from build123d import *

# Parameters (mm, degrees)
BLANKSKE_W               = 40
BLANKSKE_H               = 8.5
BLANK_DEPTH              = 10
TOOTHCUTSIM_DEPTH        = 43.09809972
TEETHCUTS_COUNT          = 14
TEETHCUTS_PITCH          = 3.14159265
BOSS_EXTRUDE1_DEPTH      = 10
SKETCH2_W                = 3
SKETCH2_H                = 3
BOSS_EXTRUDE2_DEPTH      = 60
CUT_EXTRUDE2_DEPTH       = 73.801098893
MOVE_FACE2_BY            = 5
FILLET2_R                = 8
SKETCH3_R                = 1.675
CUT_EXTRUDE1_DEPTH       = 69.738635424
SKETCH6_W                = 14.81
SKETCH6_H                = 5
BOSS_EXTRUDE3_DEPTH      = 2.5
SKETCH7_W                = 2.5
SKETCH7_H                = 5
BOSS_EXTRUDE4_DEPTH      = 5
M2_START                 = -34.81
M2_CLEARANCE_SLOT1_DEPTH = 2.5
BOSS_EXTRUDE5_DEPTH      = 5
FILLET3_R                = 5
FILLET4_R                = 1
FILLET5_R                = 0.25


with BuildPart() as part:
    # BlankSke → Blank (new body)
    with BuildSketch(Plane.XY):
        with Locations((20, 4.25)):
            Rectangle(BLANKSKE_W, BLANKSKE_H)
    extrude(amount=-BLANK_DEPTH)

    # TooCutSkeSim → ToothCutSim (cut, through all)
    with BuildSketch(Plane.XY):
        Polygon((0.44443537, 6.25), (-0.44443537, 6.25), (-1.272613241, 8.5254), (1.272613241, 8.5254), align=None)
    toothcutsim = extrude(amount=-TOOTHCUTSIM_DEPTH, mode=Mode.SUBTRACT)

    # TeethCuts: ToothCutSim ×14
    with Locations(*[(i * TEETHCUTS_PITCH, 0, 0) for i in range(1, TEETHCUTS_COUNT)]):
        add(toothcutsim, mode=Mode.SUBTRACT)

    # Sketch1 → Boss-Extrude1 (add)
    with BuildSketch(Plane.XY):
        Polygon((-20, 0), (-20, -40), (-10, -40), (-10, 0), (0, 0), (0, 6.25), (-20, 6.25), align=None)
    extrude(amount=-BOSS_EXTRUDE1_DEPTH)

    # Sketch2 → Boss-Extrude2 (add)
    with BuildSketch(Plane(origin=(40, 0, 0), x_dir=(0, 0, -1), z_dir=(1, 0, 0))):
        with Locations((-1.5, 3)):
            Rectangle(SKETCH2_W, SKETCH2_H)
    extrude(amount=-BOSS_EXTRUDE2_DEPTH)

    # Sketch5 → Cut-Extrude2 (cut, through all)
    with BuildSketch(Plane(origin=(40, 0, 0), x_dir=(0, 0, -1), z_dir=(1, 0, 0))):
        with BuildLine():
            Line((10, 2), (10, 4))
            Line((10, 4), (8, 4))
            ThreePointArc((8, 4), (7, 3), (8, 2))
            Line((8, 2), (10, 2))
        make_face()
    extrude(amount=-CUT_EXTRUDE2_DEPTH, mode=Mode.SUBTRACT)

    # Move Face2: a face moved inward by 5.0
    extrude(part.faces().sort_by_distance((-10, -20, -5))[0], amount=MOVE_FACE2_BY, dir=(-1, 0, 0), mode=Mode.SUBTRACT)

    # Fillet2
    fillet2_edges = [part.edges().sort_by_distance(p)[0] for p in [
        (-15, 0, -5),
    ]]
    fillet(fillet2_edges, radius=FILLET2_R)

    # Sketch3 → Cut-Extrude1 (cut, through all)
    with BuildSketch(Plane.ZY.offset(15)):
        with Locations((-5, -35)):
            Circle(SKETCH3_R)
    extrude(amount=CUT_EXTRUDE1_DEPTH, mode=Mode.SUBTRACT)

    # Sketch6 → Boss-Extrude3 (add)
    with BuildSketch(Plane(origin=(0, 0, -10), x_dir=(-1, 0, 0), z_dir=(0, 0, -1))):
        with Locations((27.405, -15.8)):
            Rectangle(SKETCH6_W, SKETCH6_H)
        Polygon((20, -40), (15, -40), (15, -46.25), (34.81, -46.25), (34.81, -41.25), (20, -41.25), align=None)
    extrude(amount=-BOSS_EXTRUDE3_DEPTH)

    # Sketch7 → Boss-Extrude4 (add)
    with BuildSketch(Plane.XY.offset(-7.5)):
        with Locations((-33.56, -15.8)):
            Rectangle(SKETCH7_W, SKETCH7_H)
        with Locations((-33.56, -43.75)):
            Rectangle(SKETCH7_W, SKETCH7_H)
    extrude(amount=BOSS_EXTRUDE4_DEPTH)

    # M2 Clearance Slot1: read off the stored shape, not the designer's step
    # M2 Clearance Slot1 outline → M2 Clearance Slot1 (cut)
    with BuildSketch(Plane.YZ.offset(M2_START)):
        with BuildLine():
            ThreePointArc((-44.25, -3.8), (-45.45, -5), (-44.25, -6.2))
            Line((-44.25, -6.2), (-43.25, -6.2))
            ThreePointArc((-43.25, -6.2), (-42.05, -5), (-43.25, -3.8))
            Line((-43.25, -3.8), (-44.25, -3.8))
        make_face()
        with BuildLine():
            ThreePointArc((-16.3, -3.8), (-17.5, -5), (-16.3, -6.2))
            Line((-16.3, -6.2), (-15.3, -6.2))
            ThreePointArc((-15.3, -6.2), (-14.1, -5), (-15.3, -3.8))
            Line((-15.3, -3.8), (-16.3, -3.8))
        make_face()
    extrude(amount=M2_CLEARANCE_SLOT1_DEPTH, mode=Mode.SUBTRACT)

    # M2 Clearance Slot1 2: loft between two sections, ruled curve by curve
    m2_clearance_slot1_2_from = [
        Edge.make_three_point_arc((-34.785, -43.25, -3.8), (-34.785, -42.401471863, -4.151471863), (-34.785, -42.05, -5)),
        Edge.make_three_point_arc((-34.785, -42.05, -5), (-34.785, -42.401471863, -5.848528137), (-34.785, -43.25, -6.2)),
        Edge.make_three_point_arc((-34.785, -44.25, -6.2), (-34.785, -45.098528137, -5.848528137), (-34.785, -45.45, -5)),
        Edge.make_three_point_arc((-34.785, -45.45, -5), (-34.785, -45.098528137, -4.151471863), (-34.785, -44.25, -3.8)),
        Edge.make_line((-34.785, -43.25, -6.2), (-34.785, -44.25, -6.2)),
        Edge.make_line((-34.785, -43.25, -3.8), (-34.785, -44.25, -3.8)),
    ]
    m2_clearance_slot1_2_to = [
        Edge.make_three_point_arc((-34.81, -43.25, -3.775), (-34.81, -42.383794193, -4.133794193), (-34.81, -42.025, -5)),
        Edge.make_three_point_arc((-34.81, -42.025, -5), (-34.81, -42.383794193, -5.866205807), (-34.81, -43.25, -6.225)),
        Edge.make_three_point_arc((-34.81, -44.25, -6.225), (-34.81, -45.116205807, -5.866205807), (-34.81, -45.475, -5)),
        Edge.make_three_point_arc((-34.81, -45.475, -5), (-34.81, -45.116205807, -4.133794193), (-34.81, -44.25, -3.775)),
        Edge.make_line((-34.81, -43.25, -6.225), (-34.81, -44.25, -6.225)),
        Edge.make_line((-34.81, -43.25, -3.775), (-34.81, -44.25, -3.775)),
    ]
    m2_clearance_slot1_2 = Solid(Shell([*[Face.make_surface_from_curves(m2_clearance_slot1_2_from[k], m2_clearance_slot1_2_to[k]) for k in range(6)], Face(Wire(m2_clearance_slot1_2_from)), Face(Wire(m2_clearance_slot1_2_to))]))
    add(m2_clearance_slot1_2, mode=Mode.SUBTRACT)

    # M2 Clearance Slot1 3: loft between two sections, ruled curve by curve
    m2_clearance_slot1_3_from = [
        Edge.make_three_point_arc((-34.785, -15.3, -3.8), (-34.785, -14.451471863, -4.151471863), (-34.785, -14.1, -5)),
        Edge.make_three_point_arc((-34.785, -14.1, -5), (-34.785, -14.451471863, -5.848528137), (-34.785, -15.3, -6.2)),
        Edge.make_three_point_arc((-34.785, -16.3, -6.2), (-34.785, -17.148528137, -5.848528137), (-34.785, -17.5, -5)),
        Edge.make_three_point_arc((-34.785, -17.5, -5), (-34.785, -17.148528137, -4.151471863), (-34.785, -16.3, -3.8)),
        Edge.make_line((-34.785, -15.3, -6.2), (-34.785, -16.3, -6.2)),
        Edge.make_line((-34.785, -15.3, -3.8), (-34.785, -16.3, -3.8)),
    ]
    m2_clearance_slot1_3_to = [
        Edge.make_three_point_arc((-34.81, -15.3, -3.775), (-34.81, -14.433794193, -4.133794193), (-34.81, -14.075, -5)),
        Edge.make_three_point_arc((-34.81, -14.075, -5), (-34.81, -14.433794193, -5.866205807), (-34.81, -15.3, -6.225)),
        Edge.make_three_point_arc((-34.81, -16.3, -6.225), (-34.81, -17.166205807, -5.866205807), (-34.81, -17.525, -5)),
        Edge.make_three_point_arc((-34.81, -17.525, -5), (-34.81, -17.166205807, -4.133794193), (-34.81, -16.3, -3.775)),
        Edge.make_line((-34.81, -15.3, -6.225), (-34.81, -16.3, -6.225)),
        Edge.make_line((-34.81, -15.3, -3.775), (-34.81, -16.3, -3.775)),
    ]
    m2_clearance_slot1_3 = Solid(Shell([*[Face.make_surface_from_curves(m2_clearance_slot1_3_from[k], m2_clearance_slot1_3_to[k]) for k in range(6)], Face(Wire(m2_clearance_slot1_3_from)), Face(Wire(m2_clearance_slot1_3_to))]))
    add(m2_clearance_slot1_3, mode=Mode.SUBTRACT)

    # Sketch10 → Boss-Extrude5 (add)
    with BuildSketch(Plane(origin=(-15, 0, 0), x_dir=(0, 0, -1), z_dir=(1, 0, 0))):
        Polygon((7.5, -46.25), (0, -40), (7.5, -40), align=None)
    extrude(amount=-BOSS_EXTRUDE5_DEPTH)

    # Fillet3
    fillet3_edges = [part.edges().sort_by_distance(p)[0] for p in [
        (-20, -15.8, -7.5),
        (-20, -43.75, -7.5),
    ]]
    fillet(fillet3_edges, radius=FILLET3_R)

    # Fillet4
    fillet4_edges = [part.edges().sort_by_distance(p)[0] for p in [
        (-20, -18.3, -6.25),
        (-20, -13.3, -6.25),
        (-20, -41.25, -6.25),
    ]]
    fillet(fillet4_edges, radius=FILLET4_R)

    # Fillet5
    fillet5_edges = [part.edges().sort_by_distance(p)[0] for p in [
        (-34.81, -15.8, -10),
        (-34.81, -43.75, -10),
        (-32.31, -15.8, -7.5),
        (-32.31, -43.75, -7.5),
    ]]
    fillet(fillet5_edges, radius=FILLET5_R)


solid = part.part
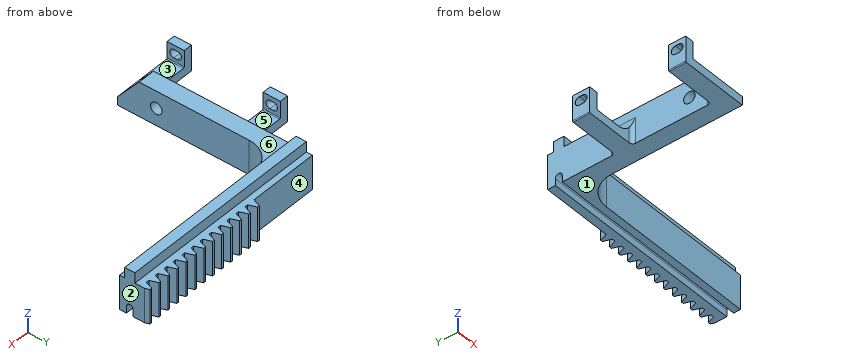
For this review, take the finished solid that the model builds, in its own axes (mm). Face numbers are marked on the shaded views. A direction names the side the tool comes from. Round coordinates to 2 decimals unless told otherwise and drop trailing zeros. Write each loop counter-clockwise with the first axis right and the second up, starting at its lowest first coordinate (ties: lowest second). Pieces come first, ordered by that corner, then holes. Notation, with made-up numbers: (38.25, 3) - (97.25, 3) arc R22 cw to (97.25, 31) - close; hole circle Ø9 at (59.5, -13). An arc over 180 degrees is marked (long way). Write item = value, one per line. Start each with the question number.
1. For the marked faces 4, 5 and 6, list the 3-axis set-ups (+Z, -Z, +X, -X, +Y, -Y) from which the entire face can be reached by the end or side of a thin tool; tool diameter is ignored.
2. Draft analysis for pull direction X (two halves, no side actions). For the marked faces 1, 2 and 3, state which applies: released by +X, released by -X, zero draft, split by the parting line, or undercut.
3. Consider section B-B on x = -17. State the section outline as (y, z) points (3 decimals), plus the area to 3 significant figures.
4. For pin 1 Ø8 at (x, y) = (-8.5, -21.5) entering from -Z; pin 2 Ø3 at (x, y) = (-33.5, -43.5) entering from +Z; pin 3 Ø5.5 at (y, z) = (-35, -5) entering from +X; pin 4 Ø2 at (x, z) = (20, 0) entering from -Y, all flat-tipped, find the tip position at first contact; note any pin that passes through.
5. Consider section A-A on y = -35. State the section outline as (x, z) points (3 decimals).
6. Consider section C-C on x = -9. State the section outline as (y, z) points, plus the area to 3 significant figures.
7. Consider section D-D on y = -28. State the section outline as (x, z) points.
8. Wall thickness on L1, parallel to Z at x = -16, y = -35 (3 decimals); L2, parallel to X at y = -32, z = -4.75; L3, parallel to X at y = -43, z = -3.5: over which ranges is each line inside the solid? List them lowest first.
Evaluation:
q1.face_4 = +Z, -Z, -X, +Y
q1.face_5 = +Z, +Y, -Y
q1.face_6 = +Z, +X, -X, -Y
q2.face_1 = zero draft
q2.face_2 = released by +X
q2.face_3 = undercut
q3.outline = (-46.25, -10) - (2, -10) - (2, -8) arc R1 cw to (4, -8) - (4, -10) - (6.25, -10) - (6.25, 0) - (4.5, 0) - (4.5, 3) - (1.5, 3) - (1.5, 0) - (-40, 0) - (-46.25, -7.5) - close; hole circle Ø3.35 at (-35, -5)
q3.area = 496 mm2
q4.pin_1 = through
q4.pin_2 = -2.5
q4.pin_3 = -15
q4.pin_4 = 0
q5.outline = (-20, -10) - (-15, -10) - (-15, -6.675) - (-20, -6.675) - close; (-20, -3.325) - (-15, -3.325) - (-15, 0) - (-20, 0) - close
q6.outline = (-0.25, -10) - (2, -10) - (2, -8) arc R1 cw to (4, -8) - (4, -10) - (6.25, -10) - (6.25, 0) - (4.5, 0) - (4.5, 3) - (1.5, 3) - (1.5, 0) - (-0.25, 0) - close
q6.area = 68.5 mm2
q7.outline = (-20, -10) - (-15, -10) - (-15, 0) - (-20, 0) - close
q8.L1 = -10 to -6.675, -3.325 to 0
q8.L2 = -20 to -15
q8.L3 = -34.81 to -32.31
